CAD build for the part. Positions are in the model's coordinates, mm. A direction names the side the tool comes from. Coordinates: 2 decimals unless noted, no trailing zeros. Write each loop counter-clockwise with the first axis right and the second up, starting at its lowest first coordinate (ties: lowest second). Pieces come first, ordered by that corner, then holes.
```python
from build123d import *

# Parameters (mm, degrees)
F0_W     = 38.1
F0_H     = 92.075
F1_DEPTH = 4.7625
F3_DEPTH = 4.7625
F5_DEPTH = 4.7625
F6_R     = 3.98907
F7_DEPTH = 55.5635


with BuildPart() as f1:
    # F0 (on Top) → F1 (new body)
    with BuildSketch(Plane.XY):
        with Locations((0, -46.0375)):
            Rectangle(F0_W, F0_H)
    extrude(amount=-F1_DEPTH)

    # F2 (on face) → F3 (join)
    with BuildSketch(Plane(origin=(-19.05, 0, 0), x_dir=(0, -1, 0), z_dir=(-1, 0, 0))):
        with BuildLine():
            Line((92.075, 0), (0, 0))
            Line((0, 0), (0, -55.5625))
            Line((0, -55.5625), (7.9375, -55.5625))
            ThreePointArc((7.9375, -55.5625), (46.0375, -17.4625), (84.1375, -55.5625))
            Line((84.1375, -55.5625), (92.075, -55.5625))
            Line((92.075, -55.5625), (92.075, 0))
        make_face()
    extrude(amount=-F3_DEPTH)

    # F4 (on face) → F5 (join)
    with BuildSketch(Plane.YZ.offset(19.05)):
        with BuildLine():
            Line((0, 0), (-92.075, 0))
            Line((-92.075, 0), (-92.075, -55.5625))
            Line((-92.075, -55.5625), (-84.1375, -55.5625))
            ThreePointArc((-84.1375, -55.5625), (-46.0375, -17.4625), (-7.9375, -55.5625))
            Line((-7.9375, -55.5625), (0, -55.5625))
            Line((0, -55.5625), (0, 0))
        make_face()
    extrude(amount=-F5_DEPTH)

    # F6 (on Top) → F7 (cut, through all)
    with BuildSketch(Plane.XY):
        with Locations((0, -14.2875)):
            Circle(F6_R)
        with Locations((0, -77.7875)):
            Circle(F6_R)
    extrude(amount=-F7_DEPTH, mode=Mode.SUBTRACT)


solid = f1.part
```
Item 1: Saw through at C-C, the plane z = -27.5. State how many separate pieces and enclosed holes the cut face has, and give its area (3 significant figures).
Item 2: Wall check: line 1 along Y through (x, z) = (0, -1.9) (3 decimals); line 2 along X through (y, z) = (-22.5, -19.5); line 3 along Z through (x, y) = (-10, -57). Give the ranges that are in metal, low to high.
Item 3: Two-plate mould, pull along X, no slides. Class faces 3 (the flat face through (14.288, -47, -13)), 4 (the flat face through (19.05, -47, -15)), 5 (the cylindrical face through (16.7, -46.88, -17.47)): +X half, -X half, draft (parallel to the pull), parting line (faces both ways), or undercut.
Item 4: Which spindle directions (+Z, -Z, +X, -X, +Y, -Y) get a long thin tool onto all of the face, cutting with end or side? Do faces 1 (the flat face through (-14.288, -45, -13)), 2 (the cylindrical face through (-16.7, -45.2, -17.47)). Say none if no direction does.
Item 5: Saw through at A-A, the plane x = 0. Write the cut outline in (y, z) (1 decimal).
Item 6: Saw through at D-D, the plane y = -80.5. Write the cut outline in (x, z), and give its area (3 significant figures).
Working result:
1. separate pieces: 4
1. enclosed holes: 0
1. area: 386 mm2
2. line 1: y = -92.075 to -81.777, -73.798 to -18.277, -10.298 to 0
2. line 2: x = -19.05 to -14.29, 14.29 to 19.05
2. line 3: z = -4.76 to 0
3. face 3: undercut
3. face 4: +X half
3. face 5: draft
4. face 1: -Z, +Y, -Y
4. face 2: -Z, +X, -X
5. outline: (-92.1, -4.8) - (-81.8, -4.8) - (-81.8, 0) - (-92.1, 0) - close; (-73.8, -4.8) - (-18.3, -4.8) - (-18.3, 0) - (-73.8, 0) - close; (-10.3, -4.8) - (0, -4.8) - (0, 0) - (-10.3, 0) - close
6. outline: (-19.05, -39.32) - (-14.29, -39.32) - (-14.29, -4.76) - (-2.92, -4.76) - (-2.92, 0) - (-19.05, 0) - close; (2.92, -4.76) - (14.29, -4.76) - (14.29, -39.32) - (19.05, -39.32) - (19.05, 0) - (2.92, 0) - close
6. area: 483 mm2
